```python
from build123d import *

# Parameters (mm, degrees)
SKETCH2_W           = 150
SKETCH2_H           = 150
BOSS_EXTRUDE1_DEPTH = 2
SKETCH3_W           = 150
SKETCH3_H           = 150
BOSS_EXTRUDE2_DEPTH = 11
SKETCH4_W           = 12
SKETCH4_H           = 12
CUT_EXTRUDE1_DEPTH  = 1


with BuildPart() as part:
    # Sketch2 → Boss-Extrude1 (new body)
    with BuildSketch(Plane.XY):
        with Locations((75, -75)):
            Rectangle(SKETCH2_W, SKETCH2_H)
    extrude(amount=BOSS_EXTRUDE1_DEPTH)

    # Sketch3 → Boss-Extrude2 (add)
    with BuildSketch(Plane.XY.offset(2)):
        with Locations((75, -75)):
            Rectangle(SKETCH3_W, SKETCH3_H)
        Polygon((147, -147), (35.571428571, -147), (35.571428571, -114.428571429), (51.525296988, -114.428571429), (51.525296988, -109.857142857), (17, -109.857142857), (17, -114.428571429), (31, -114.428571429), (31, -147), (3, -147), (3, -133), (17, -133), (17, -128.428571429), (3, -128.428571429), (3, -95.857142857), (35.571428571, -95.857142857), (35.571428571, -91.285714286), (21.571428571, -91.285714286), (21.571428571, -72.714285714), (17, -72.714285714), (17, -91.285714286), (3, -91.285714286), (3, -58.714285714), (35.571428571, -58.714285714), (35.571428571, -77.285714286), (40.142857143, -77.285714286), (40.142857143, -58.714285714), (58.714285714, -58.714285714), (58.714285714, -77.285714286), (63.285714286, -77.285714286), (63.285714286, -58.714285714), (114.428571429, -58.714285714), (114.428571429, -54.142857143), (63.285714286, -54.142857143), (63.285714286, -21.571428571), (114.428571429, -21.571428571), (114.428571429, -17), (58.714285714, -17), (58.714285714, -54.142857143), (3, -54.142857143), (3, -21.571428571), (21.571428571, -21.571428571), (21.571428571, -35.571428571), (17, -35.571428571), (17, -40.142857143), (26.142857143, -40.142857143), (26.142857143, -17), (3, -17), (3, -3), (40.142857143, -3), (40.142857143, -40.142857143), (44.714285714, -40.142857143), (44.714285714, -3), (128.428571429, -3), (128.428571429, -35.571428571), (77.285714286, -35.571428571), (77.285714286, -40.142857143), (133, -40.142857143), (133, -3), (147, -3), (147, -54.142857143), (128.428571429, -54.142857143), (128.428571429, -58.714285714), (147, -58.714285714), (147, -128.428571429), (133, -128.428571429), (133, -72.714285714), (95.857142857, -72.714285714), (95.857142857, -77.285714286), (128.428571429, -77.285714286), (128.428571429, -91.285714286), (81.857142857, -91.285714286), (81.857142857, -72.714285714), (77.285714286, -72.714285714), (77.285714286, -91.285714286), (49.571428571, -91.285714286), (49.571428571, -95.857142857), (128.428571429, -95.857142857), (128.428571429, -109.857142857), (65.525296988, -109.857142857), (65.525296988, -128.428571429), (49.571428571, -128.428571429), (49.571428571, -133), (114.428571429, -133), (114.428571429, -128.428571429), (70.09672556, -128.428571429), (70.09672556, -114.428571429), (128.428571429, -114.428571429), (128.428571429, -133), (147, -133), align=None, mode=Mode.SUBTRACT)
    extrude(amount=BOSS_EXTRUDE2_DEPTH)

    # Sketch4 → Cut-Extrude1 (cut)
    with BuildSketch(Plane.XY.offset(2)):
        with Locations((10, -10)):
            Rectangle(SKETCH4_W, SKETCH4_H)
        with Locations((140, -140)):
            Rectangle(SKETCH4_W, SKETCH4_H)
    extrude(amount=-CUT_EXTRUDE1_DEPTH, mode=Mode.SUBTRACT)


solid = part.part
```
Input: part model. Units: mm. Frame: model coordinates. Give positions to 0.01 mm unless a question says otherwise; leave off trailing zeros. Order: outer loops, then holes, each group sorted by start corner. A loop starts at its lowest first (then second) coordinate and runs counter-clockwise, first axis right, second up. Notation, with made-up numbers: (-25, -35) - (-17, -35) arc R34 cw to (-17, 3) - close; hole circle Ø10 at (85.5, 86.25). An arc over 180 degrees is marked (long way). Use a Markdown table: item, result.
(1) Draft query along Y for faces 1 (the flat face through (138, -58.714, 7)), 2 (the flat face through (150, -76, 6)). Return one class per face: released by +Y, released by -Y, zero draft, split by the parting line, or undercut.
Computed values:
| item | result |
|---|---|
| face 1 | undercut |
| face 2 | zero draft |
(2) Section query A-A (y = -75). Output: boundary loops of the cut face in (x, z), then the cut area to 3 significant figures.
Computed values:
| item | result |
|---|---|
| outline | (0, 0) - (150, 0) - (150, 13) - (147, 13) - (147, 2) - (133, 2) - (133, 13) - (95.86, 13) - (95.86, 2) - (81.86, 2) - (81.86, 13) - (77.29, 13) - (77.29, 2) - (63.29, 2) - (63.29, 13) - (58.71, 13) - (58.71, 2) - (40.14, 2) - (40.14, 13) - (35.57, 13) - (35.57, 2) - (21.57, 2) - (21.57, 13) - (17, 13) - (17, 2) - (3, 2) - (3, 13) - (0, 13) - close |
| area | 976 mm2 |
(3) Line query: line 1 (X direction, y = -16, z = 9.5); line 2 (Y direction, x = 67.5, z = 11); line 3 (Y direction, x = 123.5, z = 7.75). Output: solid intervals per line, ascending. Write a range as from..to.
Computed values:
| item | result |
|---|---|
| line 1 | x = 0..3, 40.14..44.71, 128.43..133, 147..150 |
| line 2 | y = -150..-147, -133..-109.86, -95.86..-91.29, -58.71..-54.14, -21.57..-17, -3..0 |
| line 3 | y = -150..-147, -114.43..-109.86, -95.86..-91.29, -77.29..-72.71, -40.14..-35.57, -3..0 |
(4) Section query D-D (x = 54). Output: boundary loops of the cut face in (y, z), then the cut area to 3 significant figures.
Computed values:
| item | result |
|---|---|
| outline | (-150, 0) - (0, 0) - (0, 13) - (-3, 13) - (-3, 2) - (-54.14, 2) - (-54.14, 13) - (-58.71, 13) - (-58.71, 2) - (-91.29, 2) - (-91.29, 13) - (-95.86, 13) - (-95.86, 2) - (-128.43, 2) - (-128.43, 13) - (-133, 13) - (-133, 2) - (-147, 2) - (-147, 13) - (-150, 13) - close |
| area | 517 mm2 |
(5) Section query B-B (x = 10). Output: boundary loops of the cut face in (y, z).
Computed values:
| item | result |
|---|---|
| outline | (-150, 0) - (0, 0) - (0, 13) - (-3, 13) - (-3, 2) - (-4, 2) - (-4, 1) - (-16, 1) - (-16, 2) - (-17, 2) - (-17, 13) - (-21.57, 13) - (-21.57, 2) - (-54.14, 2) - (-54.14, 13) - (-58.71, 13) - (-58.71, 2) - (-91.29, 2) - (-91.29, 13) - (-95.86, 13) - (-95.86, 2) - (-128.43, 2) - (-128.43, 13) - (-133, 13) - (-133, 2) - (-147, 2) - (-147, 13) - (-150, 13) - close |
(6) Section query C-C (y = -44.5). Output: boundary loops of the cut face in (x, z), then the cut area to 3 significant figures.
Computed values:
| item | result |
|---|---|
| outline | (0, 0) - (150, 0) - (150, 13) - (147, 13) - (147, 2) - (63.29, 2) - (63.29, 13) - (58.71, 13) - (58.71, 2) - (3, 2) - (3, 13) - (0, 13) - close |
| area | 416 mm2 |
(7) Pin query (flat end, axial travel): pin 1 (10 mm diameter, centred on x = 16.5, y = -101.5, fed in from +Z). Return the tip coordinate at first contact, or that it passes through.
Computed values:
| item | result |
|---|---|
| pin 1 | stops at z = 2 |
